The listing builds one solid part. Answer for the finished solid, in the listing's coordinates (mm). Face numbers are marked on the shaded views. A direction names the side the tool comes from. Coordinates: 2 decimals unless noted, no trailing zeros. Order: outer loops, then holes, each group sorted by start corner. A loop starts at its lowest first (then second) coordinate and runs counter-clockwise, first axis right, second up.
from build123d import *

# Parameters (mm, degrees)
F0_R     = 6
F1_DEPTH = 25
F2_R     = 5
F3_DEPTH = 25


# Not quite as in the source:
# - a feature names something its author has since deleted; it is built from what else it names


with BuildPart() as f1:
    # F0 (on Front) → F1 (new body, symmetric)
    with BuildSketch(Plane.XZ):
        with BuildLine():
            ThreePointArc((6.7823299831, 9.5), (10.9779124789, 14.0220875211), (12.5, 20))
            ThreePointArc((12.5, 20), (0, 32.5), (-12.5, 20))
            ThreePointArc((-12.5, 20), (-10.9779124789, 14.0220875211), (-6.7823299831, 9.5))
            Line((-6.7823299831, 9.5), (6.7823299831, 9.5))
        make_face()
        with Locations((0, 20)):
            Circle(F0_R, mode=Mode.SUBTRACT)
        with BuildLine():
            Line((12.5, 9.5), (12.5, 20))
            ThreePointArc((12.5, 20), (10.9779124789, 14.0220875211), (6.7823299831, 9.5))
            Line((6.7823299831, 9.5), (12.5, 9.5))
        make_face()
        with BuildLine():
            ThreePointArc((-6.7823299831, 9.5), (-10.9779124789, 14.0220875211), (-12.5, 20))
            Line((-12.5, 20), (-12.5, 9.5))
            Line((-12.5, 9.5), (-6.7823299831, 9.5))
        make_face()
    extrude(amount=F1_DEPTH, both=True)

    # F2 (on Right) → F3 (join, symmetric)
    with BuildSketch(Plane.YZ):
        with BuildLine():
            ThreePointArc((-6.7823299831, 9.5), (-10.9779124789, 4.9779124789), (-12.5, -1))
            ThreePointArc((-12.5, -1), (0, -13.5), (12.5, -1))
            ThreePointArc((12.5, -1), (10.9779124789, 4.9779124789), (6.7823299831, 9.5))
            Line((6.7823299831, 9.5), (-6.7823299831, 9.5))
        make_face()
        with Locations((0, -1)):
            Circle(F2_R, mode=Mode.SUBTRACT)
        with BuildLine():
            Line((-12.5, 9.5), (-12.5, -1))
            ThreePointArc((-12.5, -1), (-10.9779124789, 4.9779124789), (-6.7823299831, 9.5))
            Line((-6.7823299831, 9.5), (-12.5, 9.5))
        make_face()
        with BuildLine():
            ThreePointArc((6.7823299831, 9.5), (10.9779124789, 4.9779124789), (12.5, -1))
            Line((12.5, -1), (12.5, 9.5))
            Line((12.5, 9.5), (6.7823299831, 9.5))
        make_face()
    extrude(amount=F3_DEPTH, both=True)


solid = f1.part
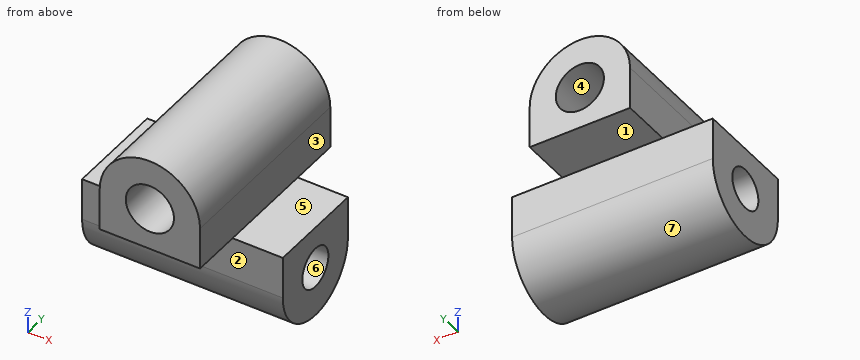
1) Each of these flat-tipped pins is pushed along its axis until it touches: P1, Ø3, axis at x = 6, y = -12, coming from the -Z side; P2, Ø12, axis at y = -7, z = 26.5, coming from the -X side; P3, Ø10, axis at x = 15.5, y = 6, coming from the +Z side; P4, Ø9, axis at y = 0, z = -1, coming from the +X side. Where does it stop, or does it pass through?
2) Determine the mould class of the marked faces 4, 5, 6 and 7 for opening direction Z: released by +Z, released by -Z, zero draft, split by the parting line, or undercut.
3) Consider L1, parallel to Z at x = 0, y = 0; L2, parallel to Z at x = 0, y = 3; L3, parallel to X at y = 16, z = 16.5. Determine where each line is inside the solid, lowest interval first.
4) A tool of negligible diameter and unlimited length cuts with its end or side. For the marked faces 1, 2 and 3, from which of +Z, -Z, +X, -X, +Y, -Y can it reach the whole face along a straight path? Write none if from no direction.
5) Section A-A (x = 0) is taken. Give the vertices of the cut face in (y, z), then the cut area to 3 significant figures.
6) Section C-C (z = 1.5) is taken. Give the vertices of the cut face in (x, y), then the cut area to 3 significant figures.
7) Section D-D (y = 19) is taken. Give the vertices of the cut face in (x, z), then the cut area to 3 significant figures.
8) Section B-B (y = 0) is taken. Give the vertices of the cut face in (x, z).
Filled sheet:
1. P1: stops at z = -7.78
1. P2: stops at x = -12.49
1. P3: stops at z = 26.78
1. P4: passes through
2. face 4: undercut
2. face 5: released by +Z
2. face 6: undercut
2. face 7: released by -Z
3. L1: z = -13.5 to -6, 4 to 14, 26 to 32.5
3. L2: z = -13.13 to -5, 3 to 14, 26 to 32.5
3. L3: x = -12.5 to -4.87, 4.87 to 12.5
4. face 1: -Z, +X, -X, +Y
4. face 2: -Z, +X, -X, -Y
4. face 3: +Z, +X, +Y, -Y
5. outline: (-25, 9.5) - (-12.5, 9.5) - (-12.5, -1) arc R12.5 ccw to (12.5, -1) - (12.5, 9.5) - (25, 9.5) - (25, 14) - (-25, 14) - close; (-25, 26) - (25, 26) - (25, 32.5) - (-25, 32.5) - close; hole circle Ø10 at (0, -1)
5. area: 979 mm2
6. outline: (-25, -12.5) - (25, -12.5) - (25, -4.33) - (-25, -4.33) - close; (-25, 4.33) - (25, 4.33) - (25, 12.5) - (-25, 12.5) - close
6. area: 817 mm2
7. outline: (-12.5, 9.5) - (12.5, 9.5) - (12.5, 20) arc R12.5 ccw to (-12.5, 20) - close; hole circle Ø12 at (0, 20)
7. area: 395 mm2
8. outline: (-25, -13.5) - (25, -13.5) - (25, -6) - (-25, -6) - close; (-25, 4) - (25, 4) - (25, 9.5) - (12.5, 9.5) - (12.5, 20) arc R12.5 ccw to (-12.5, 20) - (-12.5, 9.5) - (-25, 9.5) - close; hole circle Ø12 at (0, 20)
